from build123d import *

# Parameters (mm, degrees)
SKETCH1_W           = 35
SKETCH1_H           = 30
BOSS_EXTRUDE1_DEPTH = 10
SKETCH2_R           = 7.75
CUT_EXTRUDE1_DEPTH  = 10
SKETCH3_R           = 1.65
CUT_EXTRUDE2_DEPTH  = 10


with BuildPart() as part:
    # Sketch1 → Boss-Extrude1 (new body)
    with BuildSketch(Plane.XY):
        Rectangle(SKETCH1_W, SKETCH1_H)
    extrude(amount=BOSS_EXTRUDE1_DEPTH)

    # Sketch2 → Cut-Extrude1 (cut)
    with BuildSketch(Plane.XY.offset(10)):
        Circle(SKETCH2_R)
    extrude(amount=-CUT_EXTRUDE1_DEPTH, mode=Mode.SUBTRACT)

    # Sketch3 → Cut-Extrude2 (cut)
    with BuildSketch(Plane(origin=(17.5, 0, 0), x_dir=(0, 0, -1), z_dir=(1, 0, 0))):
        with Locations((-5, 10)):
            Circle(SKETCH3_R)
        with Locations(Location((-5, -10, 0), (0, 0, 180))):
            Circle(SKETCH3_R)
    cut_extrude2 = extrude(amount=-CUT_EXTRUDE2_DEPTH, mode=Mode.SUBTRACT)

    # Mirror1: Cut-Extrude2 across plane
    add(cut_extrude2.mirror(Plane(origin=(0, 0, 0), x_dir=(0, 0, 1), z_dir=(1, 0, 0))), mode=Mode.SUBTRACT)


solid = part.part
Could you check a few things on this model? Use its own coordinates, in mm. A direction names the side the tool comes from. Round coordinates to 2 decimals unless told otherwise and drop trailing zeros. Write each loop counter-clockwise with the first axis right and the second up, starting at its lowest first coordinate (ties: lowest second). Pieces come first, ordered by that corner, then holes. Notation, with made-up numbers: (41.5, 49.5) - (74.5, 49.5) arc R16 ccw to (74.5, 55.5) - close; hole circle Ø5 at (61.5, -0.5). An arc over 180 degrees is marked (long way). Use a Markdown table: item, result.
Q1. I want a section at B-B (x = -5.5). List the corners of the cut face in (y, z) for me.
Output values:
| item | result |
|---|---|
| outline | (-15, 0) - (-5.46, 0) - (-5.46, 10) - (-15, 10) - close; (5.46, 0) - (15, 0) - (15, 10) - (5.46, 10) - close |
Q2. Please list where these lines run through material, in increasing order: L1, parallel to Y at x = -14.5, z = 5; L2, parallel to Y at x = 0, z = 5.75; L3, parallel to Z at x = 12.25, y = -10.
Output values:
| item | result |
|---|---|
| L1 | -15 to -11.65, -8.35 to 8.35, 11.65 to 15 |
| L2 | -15 to -7.75, 7.75 to 15 |
| L3 | 0 to 3.35, 6.65 to 10 |
Q3. I want a section at A-A (y = 0). List the corners of the cut face in (x, z) for me, plus the area to 3 significant figures.
Output values:
| item | result |
|---|---|
| outline | (-17.5, 0) - (-7.75, 0) - (-7.75, 10) - (-17.5, 10) - close; (7.75, 0) - (17.5, 0) - (17.5, 10) - (7.75, 10) - close |
| area | 195 mm2 |
Q4. For faces 5 (the flat face through (-7.5, -10, 5)), 6 (the flat face through (7.5, -10, 5)), 7 (the flat face through (-17.5, 0, 5)), which set-ups out of +Z, -Z, +X, -X, +Y, -Y let a thin tool reach every point of the face, with its end or its side?
Output values:
| item | result |
|---|---|
| face 5 | -X |
| face 6 | +X |
| face 7 | +Z, -Z, -X, +Y, -Y |
Q5. I want a section at D-D (y = 10). List the corners of the cut face in (x, z) for me, plus the area to 3 significant figures.
Output values:
| item | result |
|---|---|
| outline | (-17.5, 0) - (17.5, 0) - (17.5, 3.35) - (7.5, 3.35) - (7.5, 6.65) - (17.5, 6.65) - (17.5, 10) - (-17.5, 10) - (-17.5, 6.65) - (-7.5, 6.65) - (-7.5, 3.35) - (-17.5, 3.35) - close |
| area | 284 mm2 |
Q6. For pin 1 (1 mm diameter, centred on y = 10.5, z = 4.5, fed in from +X); pin 2 (1 mm diameter, centred on y = 9.5, z = 5.5, fed in from -X), each with a flat end and sliding along its axis, tell me the tip position at first contact or that it passes through.
Output values:
| item | result |
|---|---|
| pin 1 | x = 7.5 |
| pin 2 | x = -7.5 |
Q7. Thinking about a two-plate mould opening in Z: for faces 1 (the flat face through (-4, 7, 0)), 2 (the cylindrical face through (12.57, -9, 3.69)), 3 (the flat face through (-4, 7, 10)), 4 (the flat face through (0, 15, 5)), which applies, released by +Z, released by -Z, zero draft, split by the parting line, or undercut?
Output values:
| item | result |
|---|---|
| face 1 | released by -Z |
| face 2 | undercut |
| face 3 | released by +Z |
| face 4 | zero draft |
Q8. I want a section at C-C (z = 7.75). List the corners of the cut face in (x, y) for me.
Output values:
| item | result |
|---|---|
| outline | (-17.5, -15) - (17.5, -15) - (17.5, 15) - (-17.5, 15) - close; hole circle Ø15.5 at (0, 0) |
